```python
from build123d import *

# Parameters (mm, degrees)
F4_R = 5.99999


# Not quite as in the source:
# - a fillet or chamfer is up to 0.001 mm smaller than in the source, because OpenCascade refuses the exact size


with BuildPart() as f1:
    # F0 (on Front) → F1 (revolve)
    with BuildSketch(Plane.XZ):
        with BuildLine():
            Line((-7.4487626523, 0), (0, 0))
            Line((0, 0), (83.5512373477, 0))
            Line((83.5512373477, 0), (83.5512373477, 16))
            Line((83.5512373477, 16), (80.5512373477, 16))
            Line((80.5512373477, 16), (80.5512373477, 20))
            Line((80.5512373477, 20), (60.5512373477, 20))
            Line((60.5512373477, 20), (60.5512373477, 31))
            Line((60.5512373477, 31), (48.5512373477, 31))
            ThreePointArc((48.5512373477, 31), (42.5512373477, 25), (36.5512373477, 31))
            Line((36.5512373477, 31), (-7.4487626523, 31))
            Line((-7.4487626523, 31), (-7.4487626523, 0))
        make_face()
    revolve(axis=Axis((38.0512373477, 0, 0), (1, 0, 0)))

    # F2 (on Front) → F3 (revolve, cut)
    with BuildSketch(Plane.XZ):
        Polygon((-8.5385272913, 25), (-8.5385272913, 0), (90.8953762729, 0), (90.8953762729, 6), (23.9614727087, 6), (23.9614727087, 16), (15.9614727087, 16), (15.9614727087, 20), (8.9614727087, 20), (8.9614727087, 12.5), (5.9614727087, 12.5), (5.9614727087, 16), (-6.0385272913, 16), (-6.0385272913, 25), align=None)
    revolve(axis=Axis((41.1784244908, 0, 0), (-1, 0, 0)), mode=Mode.SUBTRACT)

    # F4 (radius 6 in the source; OpenCascade refuses exactly that, so slightly less here)
    f4_edges = [f1.edges().sort_by_distance(p)[0] for p in [
        (-7.448763, 0, -31),
    ]]
    fillet(f4_edges, radius=F4_R)


solid = f1.part
```
Source: CAD feature listing. Evaluate the final solid. Frame: model axes, mm. A direction names the side the tool comes from. Give positions to 0.01 mm unless a question says otherwise; leave off trailing zeros. Write each loop counter-clockwise with the first axis right and the second up, starting at its lowest first coordinate (ties: lowest second). Pieces come first, ordered by that corner, then holes.
1. Section query A-A (x = 75.5). Return the cut outline in (y, z), then the cut area to 3 significant figures.
2. Access query for faces 1 (the face through (83.551, 0, -7)), 2 (the face through (-6.754, 7.509, 23.846)), 3 (the face through (82.03, 15.62, -3.47)), 4 (the face through (17.285, -30.736, -4.036)), 5 (the face through (15.961, 13.43, 8.98)). Directions: +Z, -Z, +X, -X, +Y, -Y. A direction counts if a zero-diameter tool reaches every point of the face in a straight line with its end or side. Return the directions, or none.
3. Pull-direction query (Z, two-part tool) for faces 6 (the face through (70.411, 19.524, -4.336)), 7 (the face through (-0.12, -15.62, -3.47)), 8 (the face through (80.551, -13.43, 8.98)); classes: +Z half, -Z half, draft (parallel to the pull), parting line (faces both ways), or undercut.
4. First-contact query: pin 1 (10 mm diameter, centred on x = 51.5, z = -11, fed in from -Y); pin 2 (3 mm diameter, centred on x = 16.5, z = 2.5, fed in from -Y); pin 3 (15 mm diameter, centred on y = -3.5, z = -11, fed in from -X); pin 4 (4 mm diameter, centred on y = 11.5, z = 12.5, fed in from +X). Flat tips, straight axial feed; report the tip coordinate or a pass-through.
5. Material intervals for line 1 along Y through (x, z) = (50, 0); line 2 along Z through (x, y) = (26, -0.5); line 3 along Y through (x, z) = (12.5, 0), sorted ascending.
6. Section query B-B (x = 10.5). Return the cut outline in (y, z).
Output values:
1. outline: circle Ø40 at (0, 0); hole circle Ø12 at (0, 0)
1. area: 1,140 mm2
2. face 1: +Z, -Z, +X, +Y, -Y
2. face 2: -X
2. face 3: +X
2. face 4: +X, -X
2. face 5: none
3. face 6: parting line
3. face 7: undercut
3. face 8: draft
4. pin 1: stops at y = -30.41
4. pin 2: stops at y = -30.98
4. pin 3: stops at x = -6.04
4. pin 4: stops at x = 83.55
5. line 1: y = -31 to -6, 6 to 31
5. line 2: z = -31 to -5.98, 5.98 to 31
5. line 3: y = -31 to -20, 20 to 31
6. outline: circle Ø62 at (0, 0); hole circle Ø40 at (0, 0)
